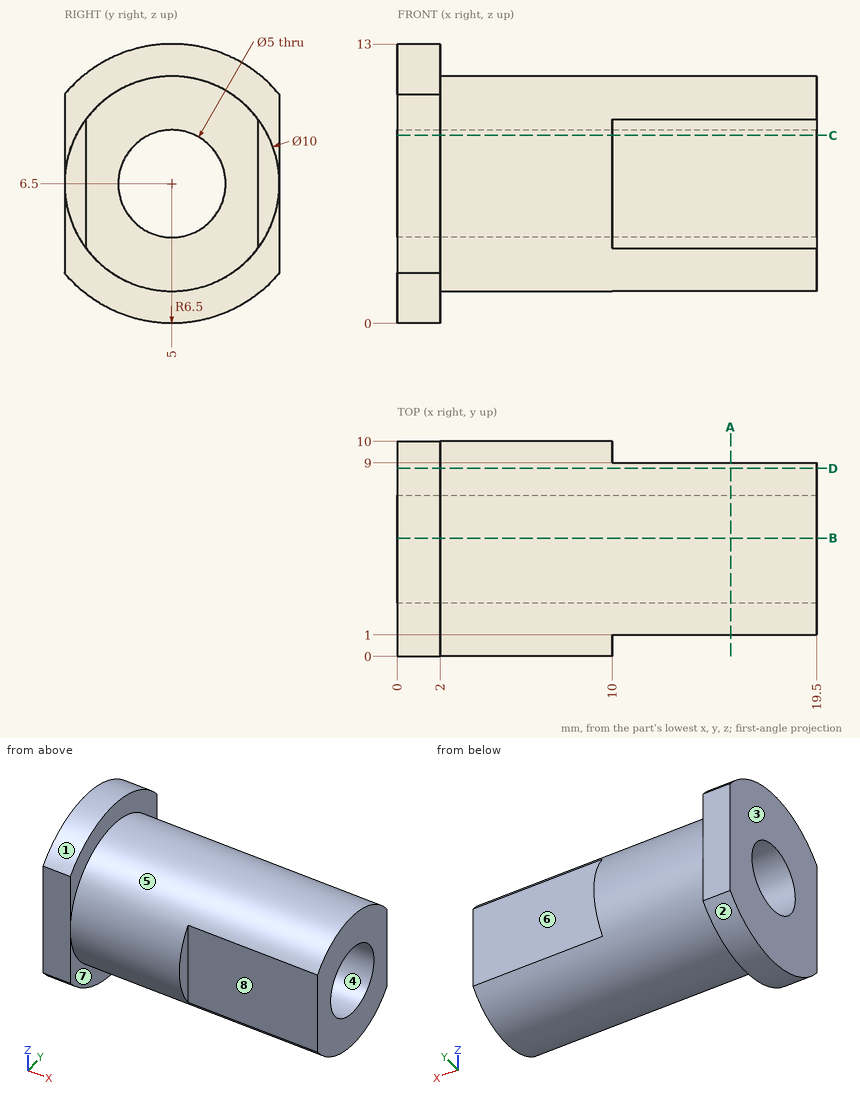
Here's the drawing with two shaded views (mm, measured from the low corner). I have some questions. A direction names the side the tool comes from. Round coordinates to 2 decimals unless told otherwise and drop trailing zeros. Loops run counter-clockwise (first coordinate to the right, second up) from the corner with the lowest first, then second, coordinate; pieces in that order, holes last. Notation, with made-up numbers: M -26.75,73.5 L -9.75,73.5 A22 ccw -9.75,109.5 Z; hole C 85,-10.75 d2. An arc over 180 degrees is marked long. Answer as a JSON object with one key per item and string values. Group by question number.
Q1. On a 3-axis mill with a long thin cutter (end or side, diameter ignored), from which of +Z, -Z, +X, -X, +Y, -Y can I reach the whole of each face in a straight line? I mean the marked faces 5, 6, 7 and 8. Say none if no direction works.
Q2. Imagine slicing it at A-A, the plane x = 15.5. Please give me the cut outline in (y, z), then the cut area to 3 significant figures.
Q3. Will these pins go through, and if not, where does the flat tip stop? pin 1 (3 mm diameter, centred on x = 15.5, z = 7, fed in from +Y); pin 2 (4 mm diameter, centred on x = 8.5, y = 2.5, fed in from +Z); pin 3 (5 mm diameter, centred on x = 6.5, y = 1, fed in from +Z).
Q4. Imagine slicing it at C-C, the plane z = 8.75. Please give me the cut outline in (x, y).
Q5. Please list where these lines run through material, in increasing order: L1, parallel to Y at x = 9.25, z = 6.5; L2, parallel to Y at x = 15.75, z = 6.5; L3, parallel to X at y = 3.25, z = 12.
Q6. We'd pull the mould along Z, two halves only. Please class the marked faces 1, 2, 3 and 4: +Z half, -Z half, draft (parallel to the pull), parting line (faces both ways), or undercut.
Q7. Imagine slicing it at D-D, the plane y = 8.75. Please give me the cut outline in (x, z).
Q8. Imagine slicing it at B-B, the plane y = 5.5. Please give me the cut outline in (x, z).
Findings:
{
 "1": {"face 5": "+X", "face 6": "+Z, -Z, +X, +Y", "face 7": "-Z, +X", "face 8": "+Z, -Z, +X, -Y"},
 "2": {"outline": "M 1,3.5 A5 ccw 9,3.5 L 9,9.5 A5 ccw 1,9.5 Z; hole C 5,6.5 d5", "area": "50.7 mm2"},
 "3": {"pin 1": "stops at y = 9", "pin 2": "stops at z = 11.47", "pin 3": "stops at z = 11.27"},
 "4": {"outline": "M 0,0 L 2,0 L 2,0.53 L 10,0.53 L 10,1 L 19.5,1 L 19.5,3.91 L 0,3.91 Z; M 0,6.09 L 19.5,6.09 L 19.5,9 L 10,9 L 10,9.47 L 2,9.47 L 2,10 L 0,10 Z"},
 "5": {"L1": "y = 0 to 2.5, 7.5 to 10", "L2": "y = 1 to 2.5, 7.5 to 9", "L3": "x = 0 to 2"},
 "6": {"face 1": "+Z half", "face 2": "-Z half", "face 3": "draft", "face 4": "undercut"},
 "7": {"outline": "M 0,1.19 L 2,1.19 L 2,3.19 L 19.5,3.19 L 19.5,9.81 L 2,9.81 L 2,11.81 L 0,11.81 Z"},
 "8": {"outline": "M 0,0.02 L 2,0.02 L 2,1.53 L 19.5,1.53 L 19.5,4.05 L 0,4.05 Z; M 0,8.95 L 19.5,8.95 L 19.5,11.47 L 2,11.47 L 2,12.98 L 0,12.98 Z"}
}
